Build history of the part. All positions in model axes, mm. Face numbers are marked on the shaded views. A direction names the side the tool comes from. Coordinates: 2 decimals unless noted, no trailing zeros. Loops run counter-clockwise (first coordinate to the right, second up) from the corner with the lowest first, then second, coordinate; pieces in that order, holes last.
Item 1: Cut at B-B (z = 5.5). List the corners of the cut face in (x, y).
Item 2: Drill centre lines: line 1 along Y through (x, z) = (14.5, 4.75); line 2 along X through (y, z) = (-7.25, 9.5); line 3 along Z through (x, y) = (-25, 8.25). Where is each one in solid material? Low to high.
Item 3: 3-axis set-ups, long thin cutter, end or side, ignore diameter. For the marked faces 1 and 2: which of +Z, -Z, +X, -X, +Y, -Y reach the whole face in a straight line?
Item 4: Cut at A-A (y = 8.5). List the corners of the cut face in (x, z).
Item 5: Cut at C-C (x = -20). List the corners of the cut face in (y, z).
Item 6: Mould opens along Y. For the marked faces 3, 4 and 5 say: released by +Y, released by -Y, zero draft, split by the parting line, or undercut.
from build123d import *

# Parameters (mm, degrees)
SKETCH2_W           = 64
SKETCH2_H           = 23
BOSS_EXTRUDE1_DEPTH = 14
SKETCH3_W           = 62.4
SKETCH3_H           = 21.4
CUT_EXTRUDE1_DEPTH  = 13.2
SKETCH4_W           = 24
SKETCH4_H           = 5
CUT_EXTRUDE3_DEPTH  = 67.515035894


with BuildPart() as part:
    # Sketch2 → Boss-Extrude1 (new body)
    with BuildSketch(Plane.XY):
        Rectangle(SKETCH2_W, SKETCH2_H)
    extrude(amount=BOSS_EXTRUDE1_DEPTH)

    # Sketch3 → Cut-Extrude1 (cut)
    with BuildSketch(Plane.XY.offset(14)):
        Rectangle(SKETCH3_W, SKETCH3_H)
    extrude(amount=-CUT_EXTRUDE1_DEPTH, mode=Mode.SUBTRACT)

    # Sketch4 → Cut-Extrude3 (cut, through all)
    with BuildSketch(Plane(origin=(32, 0, 0), x_dir=(0, 0, -1), z_dir=(1, 0, 0))):
        with Locations((-14, 0)):
            Rectangle(SKETCH4_W, SKETCH4_H)
    extrude(amount=-CUT_EXTRUDE3_DEPTH, mode=Mode.SUBTRACT)


solid = part.part
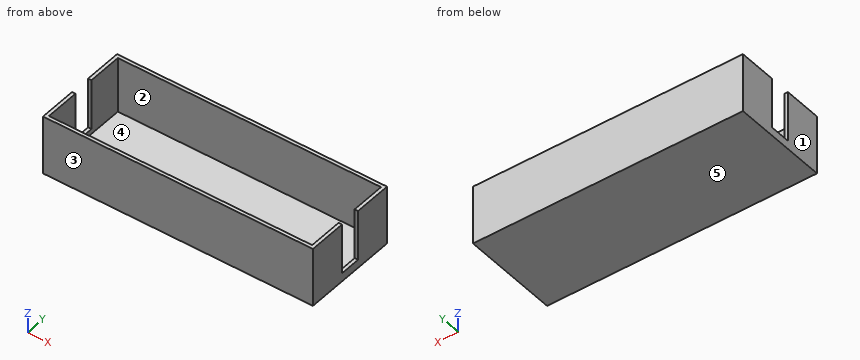
Filled sheet:
1. outline: (-32, -11.5) - (32, -11.5) - (32, -2.5) - (31.2, -2.5) - (31.2, -10.7) - (-31.2, -10.7) - (-31.2, -2.5) - (-32, -2.5) - close; (-32, 2.5) - (-31.2, 2.5) - (-31.2, 10.7) - (31.2, 10.7) - (31.2, 2.5) - (32, 2.5) - (32, 11.5) - (-32, 11.5) - close
2. line 1: y = -11.5 to -10.7, 10.7 to 11.5
2. line 2: x = -32 to -31.2, 31.2 to 32
2. line 3: z = 0 to 0.8
3. face 1: +Z, -Z, -X, +Y, -Y
3. face 2: +Z
4. outline: (-32, 0) - (32, 0) - (32, 14) - (31.2, 14) - (31.2, 0.8) - (-31.2, 0.8) - (-31.2, 14) - (-32, 14) - close
5. outline: (-11.5, 0) - (11.5, 0) - (11.5, 14) - (10.7, 14) - (10.7, 0.8) - (-10.7, 0.8) - (-10.7, 14) - (-11.5, 14) - close
6. face 3: released by -Y
6. face 4: undercut
6. face 5: zero draft
